from build123d import *

# Parameters (mm, degrees)
ESQUISSE1_R        = 2.75
ESQUISSE1_R_2      = 1.5
BOSS_EXTRU_1_DEPTH = 3
SKETCH1_R          = 1.6
CUT_EXTRUDE9_DEPTH = 10


with BuildPart() as part:
    # Esquisse1 → Boss.-Extru.1 (new body)
    with BuildSketch(Plane(origin=(0, 0, 0), x_dir=(1, 0, 0), z_dir=(0, 1, 0))):
        with BuildLine():
            Line((-145, 87.5), (155, 87.5))
            Line((155, 87.5), (155, -77.5))
            ThreePointArc((155, -77.5), (152.071067812, -84.571067812), (145, -87.5))
            Line((145, -87.5), (-145, -87.5))
            ThreePointArc((-145, -87.5), (-152.071067812, -84.571067812), (-155, -77.5))
            Line((-155, -77.5), (-155, 77.5))
            ThreePointArc((-155, 77.5), (-152.071067812, 84.571067812), (-145, 87.5))
        make_face()
        with Locations(Location((81.78624341, 76, 0), (0, 0, 270))):
            Circle(ESQUISSE1_R, mode=Mode.SUBTRACT)
        with Locations(Location((97.920945316, 58.728751177, 0), (0, 0, 270))):
            Circle(ESQUISSE1_R_2, mode=Mode.SUBTRACT)
        with Locations(Location((-148.535533906, 80.692777163, 0), (0, 0, 270))):
            Circle(ESQUISSE1_R, mode=Mode.SUBTRACT)
        with Locations(Location((-148.535533906, -81.035533906, 0), (0, 0, 270))):
            Circle(ESQUISSE1_R, mode=Mode.SUBTRACT)
        with Locations(Location((146.920945316, 58.728751177, 0), (0, 0, 270))):
            Circle(ESQUISSE1_R_2, mode=Mode.SUBTRACT)
        with Locations(Location((97.920945316, 0.728751177, 0), (0, 0, 270))):
            Circle(ESQUISSE1_R_2, mode=Mode.SUBTRACT)
        with Locations(Location((146.920945316, 0.728751177, 0), (0, 0, 270))):
            Circle(ESQUISSE1_R_2, mode=Mode.SUBTRACT)
        with Locations(Location((81.78624341, -76, 0), (0, 0, 270))):
            Circle(ESQUISSE1_R, mode=Mode.SUBTRACT)
        with Locations(Location((145, -77.5, 0), (0, 0, 270))):
            Circle(ESQUISSE1_R, mode=Mode.SUBTRACT)
    extrude(amount=BOSS_EXTRU_1_DEPTH)

    # Sketch1 → Cut-Extrude9 (cut)
    with BuildSketch(Plane(origin=(0, 3, 0), x_dir=(1, 0, 0), z_dir=(0, 1, 0))):
        with Locations(Location((35.668507743, 42.141960397, 0), (0, 0, 270))):
            Circle(SKETCH1_R)
        with Locations(Location((26.275656472, -47.123541034, 0), (0, 0, 270))):
            Circle(SKETCH1_R)
        with Locations(Location((-117.787345368, -48.053575675, 0), (0, 0, 270))):
            Circle(SKETCH1_R)
        with Locations(Location((-117.697345367, 45.896424322, 0), (0, 0, 270))):
            Circle(SKETCH1_R)
    extrude(amount=-CUT_EXTRUDE9_DEPTH, mode=Mode.SUBTRACT)


solid = part.part
Design review of the part built by this model. Coordinates are the model's own, in mm. Give positions to 0.01 mm unless a question says otherwise; leave off trailing zeros. Use CSV: the item, a comma, the result in double quotes. Start each with the question number.
1. Draft analysis for pull direction Z (two halves, no side actions). For faces 1 (the flat face through (2, 0, -1)), 2 (the cylindrical face through (-152.15, 1.48, -84.49)), 3 (the cylindrical face through (83.64, 1.48, 73.97)), state which applies: released by +Z, released by -Z, zero draft, split by the parting line, or undercut.
2. Insertion check: P1, Ø3, axis at x = -117.7, z = -45.9, coming from the -Y side; P2, Ø3.5, axis at x = 146.92, z = -58.73, coming from the -Y side. Each pin has a flat end and moves straight along its axis. Give the tip position at first contact, or say it passes through.
3. Wall thickness on L1, parallel to X at y = 2.5, z = 79.5; L2, parallel to Z at x = 145, y = 1.5; L3, parallel to X at y = 2.3, z = 77.5: over which ranges is each line inside the solid? List them lowest first.
Results found:
1,face 1,"zero draft"
1,face 2,"released by -Z"
1,face 3,"undercut"
2,P1,"passes through"
2,P2,"stops at y = 0"
3,L1,"x = -154.8 to -150.82, -146.25 to 143.11, 146.89 to 154.8"
3,L2,"z = -87.5 to 74.75, 80.25 to 87.5"
3,L3,"x = -155 to 79.48, 84.09 to 142.25, 147.75 to 155"
